CAD build for the part. Positions are in the model's coordinates, mm. A direction names the side the tool comes from. Coordinates: 2 decimals unless noted, no trailing zeros. Order: outer loops, then holes, each group sorted by start corner. A loop starts at its lowest first (then second) coordinate and runs counter-clockwise, first axis right, second up. Notation, with made-up numbers: M 82,-9 L 118,-9 A20 cw 118,27 Z; hole C 31,59 d7. An arc over 180 degrees is marked long. Write item = value, one per line.
Autodesk Inventor part; units mm, degrees
ref_plane "Work Plane1" through (29, 0, 0) normal (0, -1, 0) x (1, 0, 0)
ref_plane "YZ Plane" through (0, 0, 0) normal (1, 0, 0) x (0, 1, 0)
ref_plane "XZ Plane" through (0, 0, 0) normal (0, 1, 0) x (-1, 0, 0)
sketch "Skizze1" plane through (0, 0, 0) normal (0, 0, 1) x (1, 0, 0)
  line L0 (-0.5, 0) -> (5, 0)
  line L1 (5, 0) -> (5, 1)
  line L2 (5, 1) -> (1, 1)
  line L3 (1, 1) -> (0.7545, 1)
  line L4 (0.7545, 1) -> (0, 1)
  line L5 (0, 1) -> (0, 1.9)
  line L6 (0, 1.9) -> (-2, 1.9)
  line L7 (-2, 1.9) -> (-2, 0.866)
  line L8 (-2, 0.866) -> (-1, 0.866)
  line L9 (-1, 0.866) -> (-0.5, 0)
  line L10 (-3.4, 0) -> (6.4, 0)
  line L11 (0, -0.38) -> (0, 2.28)
  line L12 (1, 1) -> (0, 1) construction
  dimension "d1" = 4
  dimension "d2" = 0.2455
  dimension "d3" = 2
  dimension "d4" = 1
  dimension "d5" = 60
  dimension "d6" = 2
  dimension "d7" = 2
  dimension "d8" = 1.7321
  dimension "d9" = 3.8
  dimension "d26" = 5
revolve "Körper" add sketch "Skizze1" angle 360 about axis through (-0.5, 0, 0) along (1, 0, 0)
sketch "Skizze2" plane through (-2, 0, 0) normal (-1, 0, 0) x (0, 0, 1)
  circle A0 centre (0, 0) radius 0.866
  line L0 (0, -2.66) -> (0, 2.66)
  line L1 (-2.66, 0) -> (2.66, 0)
  line L2 (0.866, 0) -> (0.433, -0.75)
  line L3 (0.433, -0.75) -> (-0.433, -0.75)
  line L4 (-0.433, -0.75) -> (-0.866, 0)
  line L5 (-0.866, 0) -> (-0.433, 0.75)
  line L6 (-0.433, 0.75) -> (0.433, 0.75)
  line L7 (0.433, 0.75) -> (0.866, 0)
  point P0 (0, 0)
extrude "Loch" add sketch "Skizze2" against normal up to next contours L7 A0 | A0 L2 | L6 L0 A0 | A0 L0 L3 | L0 L6 A0 | A0 L3 L0 | L4 A0 | A0 L5
fillet "Rundung1" radius 0.2 1 edges at (-2, -1.9, 0)
thread "Gewinde"
chamfer "Fase1" distance 0.2454 distance2 0.2454 1 edges at (5, -1, 0) measured on face at (5, -0.4588, -0.3309)
ref_plane "Work Plane1" through (29, 0, 0) normal (0, -1, 0) x (1, 0, 0)
fillet "Fillet2" radius 0.1 1 edges at (0, -1, 0)
equation "\"d1\" = GEL"
equation "\"d3\" = KOH"
equation "\"d4\" = INTI"
equation "\"d6\" = GD"
equation "\"d7\" = BDM"
equation "\"d8\" = 1.1547 * SW"
equation "\"d9\" = KOD"
equation "\"d26\" = NLG"
equation "\"d30\" = R"
equation "\"d17\" = RR"
equation "\"d13\" = GEL"
equation "\"d15\" = -0.5 * SPD + 0.5 * GD"
equation "\"d16\" = GUL"
equation "\"GD\" = 2"
equation "\"NLG\" = 5"
equation "\"GEL\" = 4"
equation "\"KOD\" = 3.8"
equation "\"KOH\" = 2"
equation "\"INTI\" = 1"
equation "\"GAL\" = 0.61345 * PTC"
equation "\"GUL\" = 0.61345 * PTC"
equation "\"BDM\" = NND"
equation "\"SW\" = 1.5"
equation "\"RR\" = 0.2"
equation "\"SPD\" = NND - 1.2269 * PTC"
equation "\"R\" = 0.1"
equation "\"TOA\" = 30deg"
equation "\"GD1\" = THREADDIA - 1.2269 * PTC"
equation "\"THREADDIA\" = 2"
equation "\"FAWI\" = 45deg"
equation "\"PTC\" = 0.4"
equation "\"NND\" = 2"
equation "\"E0\" = 1.155 * SW"
properties part number "ISO 4762 - M2 x 5" material "Edelstahl, 440C"
(1) Wall check: line 1 (Z direction, x = -1, y = 1.55); line 2 (X direction, y = -0.8, z = 1.1); line 3 (Y direction, x = -1.25, z = -0.65). Give the ranges that are in metal, low to high. Write a range as from..to.
Evaluation:
line_1 = -1.1..1.1
line_2 = -2..0
line_3 = -1.79..-0.37, 0.37..1.79
(2) Slice it at A-A, the plane x = 0.25. Write the cut outline in (y, z).
Evaluation:
outline = C 0,0 d2
(3) Tool access for faces 1 (the face through (-1.5, 0.75, 0)), 2 (the face through (-2, 1, 0)): list every direction of +Z, -Z, +X, -X, +Y, -Y with a clear straight run to the whole face (end or side of a thin tool).
Evaluation:
face_1 = -X
face_2 = +Z, -Z, -X, +Y, -Y
(4) Pull direction Y, two halves, no side cores. Call faces 3 (the face through (-0.53, 0.05, -0.02)), 4 (the face through (2, 0, 1)), 5 (the face through (0, 1, -1)): +Y half, -Y half, draft (parallel to the pull), parting line (faces both ways), or undercut.
Evaluation:
face_3 = undercut
face_4 = parting line
face_5 = draft
(5) Pin check, flat tip, straight feed: pin 1 Ø1 at (x, z) = (1, 1) entering from +Y. Stop position of the tip, or through.
Evaluation:
pin_1 = 0.87
